For this review, take the finished solid that the model builds, in its own axes (mm). A direction names the side the tool comes from. Coordinates: 2 decimals unless noted, no trailing zeros. Order: outer loops, then holes, each group sorted by start corner. A loop starts at its lowest first (then second) coordinate and runs counter-clockwise, first axis right, second up. Notation, with made-up numbers: (65, 20.25) - (81, 20.25) arc R23 cw to (81, 58.25) - close; hole circle Ø6 at (-11.75, -8). An arc over 180 degrees is marked (long way). One line per item, written item: value. Start each with the question number.
(1) To check wall thickness, follow line 1 along Z through (x, y) = (0, 3.8); line 2 along Z through (x, y) = (0, 1.6); line 3 along X through (y, z) = (2.9, 0.25). State the ranges of each line that lie inside material, in increasing order.
(2) Clearance check with a flat-ended pin moving along its axis: pin 1 (3 mm diameter, centred on x = 0, z = -7.07, fed in from -Y). State where the tip first meets the part, or that it passes through.
(3) Consider section C-C on y = 2.8. Write out the cut boundary in (x, z).
(4) Consider section A-A on x = 0. Count the separate pieces of the cut face and the enclosed holes in it, then the cut area to 3 significant figures.
(5) Mouldability with a two-part tool opening along X and no side actions: class faces 3 (the cylindrical face through (9.443, 3.337, -2.974)), 4 (the flat face through (4, 2.1, 4)), 5 (the cylindrical face through (0.596, 2.021, 2.685)) as released by +X, released by -X, zero draft, split by the parting line, or undercut.
(6) For faces 1 (the cylindrical face through (0.27, 3.32, -5.85)), 2 (the flat face through (-1, 4.1, 1)), list the 3-axis set-ups (+Z, -Z, +X, -X, +Y, -Y) from which the entire face can be reached by the end or side of a thin tool; tool diameter is ignored.
```python
from build123d import *

# Parameters (mm, degrees)
CHAMFER_1_SIZE               = 0.3
HOLE_WIZARD_M3_1_D           = 2.5
HOLE_WIZARD_M3_1_CSINK_D     = 2.55
HOLE_WIZARD_M3_1_CSINK_ANGLE = 90
SKETCH_5_R                   = 2.75
CUT_EXTRUDE_1_DEPTH          = 1
CUT_EXTRUDE_1_DEPTH_BACK     = 4.1


with BuildPart() as part:
    # 草图2 → 旋转1 (revolve)
    with BuildSketch(Plane.XY):
        Polygon((4.95, 0), (0, 0), (0, 4.6), (9.9, 4.6), (9.9, 2.1), (4.95, 2.1), align=None)
    revolve(axis=Axis((0, 0, 0), (0, 1, 0)))

    # 倒角1
    chamfer_1_edges = [part.edges().sort_by_distance(p)[0] for p in [
        (-9.9, 4.6, 0),
        (-9.9, 2.1, 0),
        (-4.95, 0, 0),
    ]]
    chamfer(chamfer_1_edges, length=CHAMFER_1_SIZE)

    # M3 螺纹孔的螺纹孔钻头1 (through all)
    with Locations(Plane(origin=(0, 4.6, 0), x_dir=(1, 0, 0), z_dir=(0, 1, 0))):
        with Locations((7.071067812, 0), (0, -7.071067812), (-7.071067812, 0), (0, 7.071067812), (0, 0)):
            CounterSinkHole(HOLE_WIZARD_M3_1_D / 2, HOLE_WIZARD_M3_1_CSINK_D / 2, counter_sink_angle=HOLE_WIZARD_M3_1_CSINK_ANGLE)

    # 草图5 → 切除-拉伸1 (cut, two sides)
    with BuildSketch(Plane(origin=(0, 0, 0), x_dir=(-1, 0, 0), z_dir=(0, -1, 0))) as cut_extrude_1_sk:
        Circle(SKETCH_5_R)
    extrude(amount=CUT_EXTRUDE_1_DEPTH, mode=Mode.SUBTRACT)
    extrude(cut_extrude_1_sk.sketch, amount=-CUT_EXTRUDE_1_DEPTH_BACK, mode=Mode.SUBTRACT)


solid = part.part
```
Geometry check:
1. line 1: z = -9.9 to -8.32, -5.82 to -2.75, 2.75 to 5.82, 8.32 to 9.9
1. line 2: z = -4.95 to -2.75, 2.75 to 4.95
1. line 3: x = -9.9 to -8.3, -5.85 to -2.74, 2.74 to 5.85, 8.3 to 9.9
2. pin 1: stops at y = 2.1
3. outline: circle Ø19.8 at (0, 0); hole circle Ø2.5 at (-7.07, 0); hole circle Ø5.5 at (0, 0); hole circle Ø2.5 at (0, -7.07); hole circle Ø2.5 at (0, 7.07); hole circle Ø2.5 at (7.07, 0)
4. separate pieces: 4
4. enclosed holes: 0
4. area: 33.7 mm^2
5. face 3: split by the parting line
5. face 4: zero draft
5. face 5: undercut
6. face 1: +Y, -Y
6. face 2: -Y
